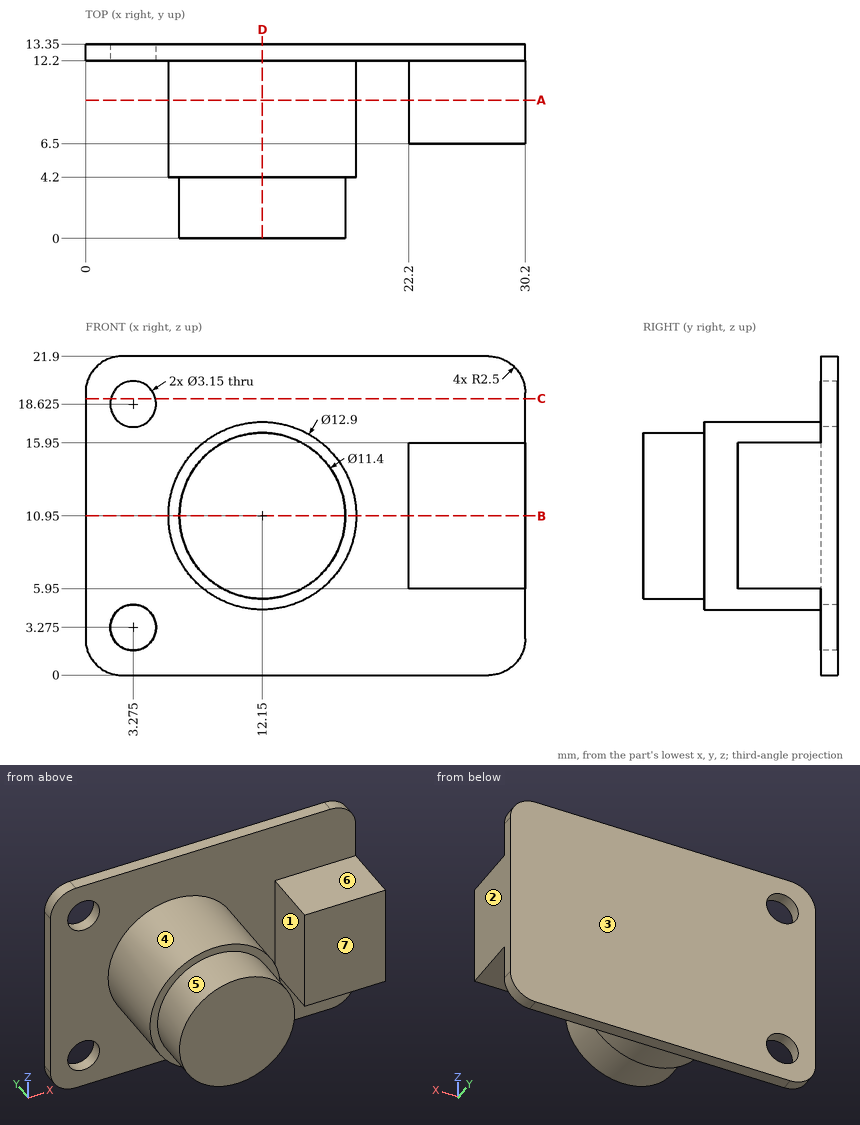
The figure shows three views and two pictorial views of one solid part (mm, origin at its lowest corner). Answer the questions. A direction names the side the tool comes from. Round coordinates to 2 decimals unless told otherwise and drop trailing zeros. Order: outer loops, then holes, each group sorted by start corner. A loop starts at its lowest first (then second) coordinate and runs counter-clockwise, first axis right, second up. Notation, with made-up numbers: M 29,15 L 66,15 A19 ccw 66,30 Z; hole C -40,68 d8. An arc over 180 degrees is marked long. Put each result on its own line as item: value. Start each with the question number.
Q1. Section C-C, the plane z = 19 is taken. Write down the section's boundary in (x, y), and give its area (3 significant figures).
Q2. Section B-B, the plane z = 10.95 is taken. Write down the section's boundary in (x, y), and give its area (3 significant figures).
Q3. Straight lines are drawn through the part: L1, parallel to Y at x = 11, z = 2.25; L2, parallel to Y at x = 25.5, z = 14; L3, parallel to X at y = 8, z = 8.5. For each, find the intervals that lie inside material, in ascending order. Write a range as [from, to].
Q4. Section A-A, the plane y = 9.5 is taken. Write down the section's boundary in (x, z).
Q5. Section D-D, the plane x = 12.15 is taken. Write down the section's boundary in (y, z), and give its area (3 significant figures).
Q6. For a pull along X with two mould halves and no side action, classify the marked faces 1, 2, 3 and 4 as pulls with the +X half, pulls with the -X half, needs draft (parallel to the pull), parting line crosses it, or undercut.
Q7. Flat-ended cylindrical pins translate along their axes: pin 1 (4.5 mm diameter, centred on x = 28, y = 8.5, fed in from -Z); pin 2 (4.5 mm diameter, centred on y = 8.5, z = 13.5, fed in from -X); pin 3 (6 mm diameter, centred on x = 15, y = 9, fed in from -Z). Find the tip coordinate at first contact, or state that the pin passes through.
Q8. A tool of negligible diameter and unlimited length cuts with its end or side. For the marked faces 5, 6 and 7, from which of +Z, -Z, +X, -X, +Y, -Y can it reach the whole face along a straight path? Write none if from no direction.
Findings below:
1. outline: M 0,12.2 L 1.75,12.2 L 1.75,13.35 L 0,13.35 Z; M 4.8,12.2 L 30.2,12.2 L 30.2,13.35 L 4.8,13.35 Z
1. area: 31.2 mm^2
2. outline: M 0,12.2 L 5.7,12.2 L 5.7,4.2 L 6.45,4.2 L 6.45,0 L 17.85,0 L 17.85,4.2 L 18.6,4.2 L 18.6,12.2 L 22.2,12.2 L 22.2,6.5 L 30.2,6.5 L 30.2,13.35 L 0,13.35 Z
2. area: 231 mm^2
3. L1: y = [12.2, 13.35]
3. L2: y = [6.5, 13.35]
3. L3: x = [6.18, 18.12], [22.2, 30.2]
4. outline: C 12.15,10.95 d12.9; M 22.2,5.95 L 30.2,5.95 L 30.2,15.95 L 22.2,15.95 Z
5. outline: M 0,5.25 L 4.2,5.25 L 4.2,4.5 L 12.2,4.5 L 12.2,0 L 13.35,0 L 13.35,21.9 L 12.2,21.9 L 12.2,17.4 L 4.2,17.4 L 4.2,16.65 L 0,16.65 Z
5. area: 176 mm^2
6. face 1: undercut
6. face 2: pulls with the +X half
6. face 3: needs draft
6. face 4: undercut
7. pin 1: stops at z = 5.95
7. pin 2: stops at x = 5.71
7. pin 3: stops at z = 4.5
8. face 5: -Y
8. face 6: +Z, +X, -Y
8. face 7: +Z, -Z, +X, -Y
